Part model, mm, in its own coordinate system. A direction names the side the tool comes from. Coordinates: 2 decimals unless noted, no trailing zeros. Loops run counter-clockwise (first coordinate to the right, second up) from the corner with the lowest first, then second, coordinate; pieces in that order, holes last. Notation, with made-up numbers: (8, 24.5) - (19, 24.5) arc R24 ccw to (19, 55.5) - close; hole circle Ø1 at (55.5, -24). An arc over 180 degrees is marked (long way). Use a Markdown table: item, result. Add a question column.
1) Band-saw the part on C-C (y = -13). Give the cut face in (x, z), plus the area to 3 significant figures.
2) Band-saw the part on A-A (x = 10). Give the cut face in (y, z).
3) Probe probe 1 along X at (y, z) = (-5, 35.5); probe 2 along Z at (x, y) = (16, -7); probe 3 along X at (y, z) = (2, 38). List the from-to ranges inside material, lowest first. Write a range as [from, to].
4) Drop a flat-ended pin along its axis: P1, Ø1, axis at x = -19, z = 6.5, coming from the +Y side. Give the stop position or say it passes through.
5) Band-saw the part on B-B (z = 37). Give the cut face in (x, y), plus the area to 3 significant figures.
6) Pull direction Z, two halves, no side cores. Call faces 1 (the face through (4.441, -15, 13)), 2 (the face through (36.573, -25, 7)), 3 (the face through (16, -14, 0)): +Z half, -Z half, draft (parallel to the pull), parting line (faces both ways), or undercut.
7) Band-saw the part on D-D (z = 19). Give the cut face in (x, y).
8) Tool access for faces 4 (the face through (28.441, -15, 13)), 5 (the face through (-3.427, -25, 7)), 6 (the face through (49.391, -17.146, 40.643)): list every direction of +Z, -Z, +X, -X, +Y, -Y with a clear straight run to the whole face (end or side of a thin tool).
from build123d import *

# Parameters (mm, degrees)
F0_W      = 40
F0_H      = 46
F1_DEPTH  = 46
F3_W      = 24
F3_H      = 30
F4_DEPTH  = 46
F5_R      = 18
F6_DEPTH  = 26
F7_R      = 18
F8_DEPTH  = 26
F9_R      = 9
F10_DEPTH = 92


with BuildPart() as f1:
    # F0 (on Top) → F1 (new body)
    with BuildSketch(Plane.XY):
        with Locations((16.572512, -14.664019)):
            Rectangle(F0_W, F0_H)
    extrude(amount=F1_DEPTH)

    # F3 (on face) → F4 (cut)
    with BuildSketch(Plane.XZ.offset(37.664019)):
        with Locations((16.440791, 23.289474)):
            Rectangle(F3_W, F3_H)
    extrude(amount=-F4_DEPTH, mode=Mode.SUBTRACT)

    # F5 (on face) → F6 (join)
    with BuildSketch(Plane.YZ.offset(36.572512)):
        with Locations((-14.802633, 22.796053)):
            Circle(F5_R)
    extrude(amount=F6_DEPTH)

    # F7 (on face) → F8 (join)
    with BuildSketch(Plane(origin=(-3.427488, 0, 0), x_dir=(0, -1, 0), z_dir=(-1, 0, 0))):
        with Locations((14.802634, 23)):
            Circle(F7_R)
    extrude(amount=F8_DEPTH)

    # F9 (on face) → F10 (cut)
    with BuildSketch(Plane(origin=(-29.427488, 0, 0), x_dir=(0, -1, 0), z_dir=(-1, 0, 0))):
        with Locations((14.802634, 23)):
            Circle(F9_R)
    extrude(amount=-F10_DEPTH, mode=Mode.SUBTRACT)


solid = f1.part
Answer block:
| question | item | result |
|---|---|---|
| 1 | outline | (-29.43, 5.09) - (-3.43, 5.09) - (-3.43, 0) - (36.57, 0) - (36.57, 4.89) - (62.57, 4.89) - (62.57, 14.18) - (28.44, 14.18) - (28.44, 8.29) - (4.44, 8.29) - (4.44, 14.18) - (-29.43, 14.18) - close; (-29.43, 31.82) - (4.44, 31.82) - (4.44, 38.29) - (28.44, 38.29) - (28.44, 31.82) - (62.57, 31.82) - (62.57, 40.71) - (36.57, 40.71) - (36.57, 46) - (-3.43, 46) - (-3.43, 40.91) - (-29.43, 40.91) - close |
| 1 | area | 1,780 mm2 |
| 2 | outline | (-37.66, 0) - (8.34, 0) - (8.34, 8.29) - (-37.66, 8.29) - close; (-37.66, 38.29) - (8.34, 38.29) - (8.34, 46) - (-37.66, 46) - close |
| 3 | probe 1 | [-29.43, 4.44], [28.44, 62.57] |
| 3 | probe 2 | [0, 8.29], [38.29, 46] |
| 3 | probe 3 | [-3.43, 4.44], [28.44, 36.57] |
| 4 | P1 | y = -6.56 |
| 5 | outline | (-29.43, -26.12) - (-3.43, -26.12) - (-3.43, -37.66) - (4.44, -37.66) - (4.44, 8.34) - (-3.43, 8.34) - (-3.43, -3.49) - (-29.43, -3.49) - close; (28.44, -37.66) - (36.57, -37.66) - (36.57, -25.86) - (62.57, -25.86) - (62.57, -3.75) - (36.57, -3.75) - (36.57, 8.34) - (28.44, 8.34) - close |
| 5 | area | 1,900 mm2 |
| 6 | face 1 | undercut |
| 6 | face 2 | draft |
| 6 | face 3 | -Z half |
| 7 | outline | (-29.43, -32.35) - (-3.43, -32.35) - (-3.43, -37.66) - (4.44, -37.66) - (4.44, -22.86) - (-29.43, -22.86) - close; (-29.43, -6.74) - (4.44, -6.74) - (4.44, 8.34) - (-3.43, 8.34) - (-3.43, 2.75) - (-29.43, 2.75) - close; (28.44, -37.66) - (36.57, -37.66) - (36.57, -32.4) - (62.57, -32.4) - (62.57, -22.86) - (28.44, -22.86) - close; (28.44, -6.74) - (62.57, -6.74) - (62.57, 2.79) - (36.57, 2.79) - (36.57, 8.34) - (28.44, 8.34) - close |
| 8 | face 4 | +Y, -Y |
| 8 | face 5 | -X |
| 8 | face 6 | +X |
